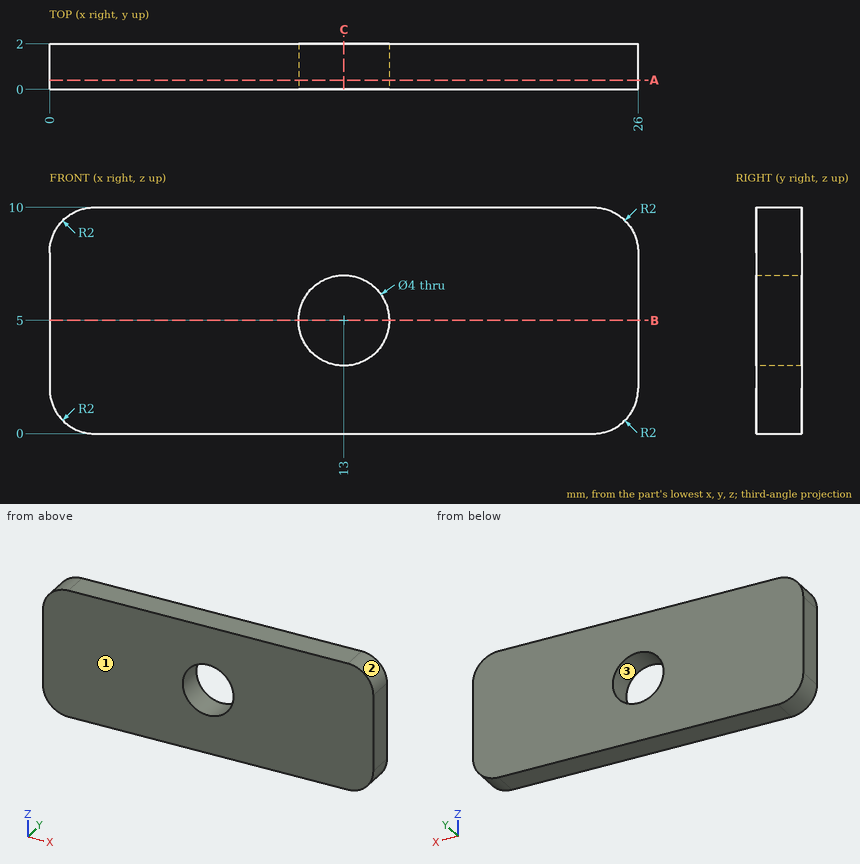
Input: dimensioned drawing with shaded views. Units: mm. Origin: part minimum x, y, z. Round coordinates to 2 decimals unless told otherwise and drop trailing zeros. Loops run counter-clockwise (first coordinate to the right, second up) from the corner with the lowest first, then second, coordinate; pieces in that order, holes last. Notation, with made-up numbers: M 44.5,41 L 49.5,41 A4 cw 49.5,46 Z; hole C 66.25,-32.75 d9. An arc over 180 degrees is marked long. Answer in a Markdown table with one row per item. Add a question column.
1. Section A-A (y = 0.4). Output: boundary loops of the cut face in (x, z), and give its area (3 significant figures).
2. Section C-C (x = 13). Output: boundary loops of the cut face in (y, z).
3. Ray query, probe 1 along X at (y, z) = (1.4, 5); probe 2 along X at (y, z) = (1.4, 4); probe 3 along X at (y, z) = (0.3, 9). Return the intervals inside material, ascending.
4. Mould query, pull axis Z, two halves, no side actions, for the marked faces 1, 2 and 3. Classes: released by +Z, released by -Z, zero draft, split by the parting line, or undercut.
5. Section B-B (z = 5). Output: boundary loops of the cut face in (x, y).
Values follow:
| question | item | result |
|---|---|---|
| 1 | outline | M 0,2 A2 ccw 2,0 L 24,0 A2 ccw 26,2 L 26,8 A2 ccw 24,10 L 2,10 A2 ccw 0,8 Z; hole C 13,5 d4 |
| 1 | area | 244 mm^2 |
| 2 | outline | M 0,0 L 2,0 L 2,3 L 0,3 Z; M 0,7 L 2,7 L 2,10 L 0,10 Z |
| 3 | probe 1 | 0 to 11, 15 to 26 |
| 3 | probe 2 | 0 to 11.27, 14.73 to 26 |
| 3 | probe 3 | 0.27 to 25.73 |
| 4 | face 1 | zero draft |
| 4 | face 2 | released by +Z |
| 4 | face 3 | undercut |
| 5 | outline | M 0,0 L 11,0 L 11,2 L 0,2 Z; M 15,0 L 26,0 L 26,2 L 15,2 Z |
